Input: part model. Units: mm. Frame: model coordinates. A direction names the side the tool comes from. Round coordinates to 2 decimals unless told otherwise and drop trailing zeros. Order: outer loops, then holes, each group sorted by start corner. A loop starts at its lowest first (then second) coordinate and runs counter-clockwise, first axis right, second up. Notation, with made-up numbers: (86, 71.5) -> (106, 71.5) arc R20 ccw to (106, 100.5) -> close; hole circle Ø4 at (18, 0). An arc over 180 degrees is marked (long way). Use a Markdown table: item, result.
Autodesk Inventor part; units mm, degrees
ref_plane "YZ Plane" through (0, 0, 0) normal (1, 0, 0) x (0, 1, 0)
ref_plane "XZ Plane" through (0, 0, 0) normal (0, 1, 0) x (-1, 0, 0)
ref_plane "XY Plane" through (0, 0, 0) normal (0, 0, 1) x (1, 0, 0)
sketch "スケッチ1" plane through (0, 0, 0) normal (0, 0, 1) x (1, 0, 0)
  circle A0 centre (0, 0) radius 2
  dimension "d0" = 4
extrude "押し出し1" add sketch "スケッチ1" along normal blind 6
sketch "スケッチ2" plane through (0, 0, 6) normal (0, 0, 1) x (1, 0, 0)
  circle A0 centre (0, 0) radius 2
  circle A1 centre (0, 0) radius 4
  dimension "d3" = 8
extrude "押し出し2" add sketch "スケッチ2" along normal blind 3 contours A0 | A1
fillet "フィレット1" radius 3 1 edges at (-4, 0, 9)
thread "ねじ1"
sketch "スケッチ3" plane through (0, 0, 0) normal (0, 0, -1) x (-1, 0, 0)
  circle A0 centre (0, 0) radius 2
extrude "押し出し3" add sketch "スケッチ3" along normal blind 9
properties part number "SB　M4 15mm なべネジ" material "Stainless Steel, 440C"
1) Contact query for flat-ended pins moving along their axis: P1, Ø2, axis at x = -0.5, z = 4.5, coming from the +Y side; P2, Ø1.5, axis at x = -0.5, z = -5, coming from the -Y side; P3, Ø4, axis at x = 2, y = -2, coming from the -Z side; P4, Ø1.5, axis at x = 3, y = -0.5, coming from the +Z side. Output: stop coordinate, or through.
Answer key:
| item | result |
|---|---|
| P1 | stops at y = 2 |
| P2 | stops at y = -2 |
| P3 | stops at z = -9 |
| P4 | stops at z = 8.71 |
2) Ray query, probe 1 along Y at (x, z) = (0, -3); probe 2 along X at (y, z) = (1.75, -5.25); probe 3 along Z at (x, y) = (0.75, -2.5). Return the intervals inside material, ascending.
Answer key:
| item | result |
|---|---|
| probe 1 | y = -2 to 2 |
| probe 2 | x = -0.97 to 0.97 |
| probe 3 | z = 6 to 8.53 |
3) Set-up query: faces 1 (the face through (-2, -1, 6)), 2 (the face through (0, 0, 9)). Return all of +Z, -Z, +X, -X, +Y, -Y with unobstructed straight access to the full face (end or side cutting, diameter ignored); none if empty.
Answer key:
| item | result |
|---|---|
| face 1 | -Z |
| face 2 | +Z, +X, -X, +Y, -Y |
4) Cut plane A-A on z = -1. Return loops of the section in (x, y), and give its area (3 significant figures).
Answer key:
| item | result |
|---|---|
| outline | circle Ø4 at (0, 0) |
| area | 12.6 mm^2 |
